```python
from build123d import *

# Parameters (mm, degrees)
SKETCH1_W           = 21.59
SKETCH1_H           = 16.51
SKETCH1_R           = 0.5
SKETCH1_W_2         = 15.24
SKETCH1_H_2         = 10.16
SKETCH1_W_3         = 9.2075
SKETCH1_H_3         = 2.38125
BOSS_EXTRUDE1_DEPTH = 1.5875
SKETCH1_3_W         = 15.24
SKETCH1_3_H         = 10.16
BOSS_EXTRUDE2_DEPTH = 3.175


with BuildPart() as part:
    # Sketch1 → Boss-Extrude1 (new body)
    # profile 1 of 4: a face of its own
    with BuildSketch(Plane.XY):
        Rectangle(SKETCH1_W, SKETCH1_H)
        with Locations((0, 7.46125)):
            Circle(SKETCH1_R, mode=Mode.SUBTRACT)
        with Locations((0, -7.46125)):
            Circle(SKETCH1_R, mode=Mode.SUBTRACT)
        Rectangle(SKETCH1_W_2, SKETCH1_H_2, mode=Mode.SUBTRACT)
    # profile 2 of 4: a face of its own
    with BuildSketch(Plane.XY):
        Rectangle(SKETCH1_W_2, SKETCH1_H_2)
    # profile 3 of 4: a face of its own
    with BuildSketch(Plane.XY):
        with Locations((0, 9.445625)):
            Rectangle(SKETCH1_W_3, SKETCH1_H_3)
    # profile 4 of 4: a face of its own
    with BuildSketch(Plane.XY):
        with Locations((0, -9.445625)):
            Rectangle(SKETCH1_W_3, SKETCH1_H_3)
    extrude(amount=BOSS_EXTRUDE1_DEPTH)

    # Sketch1_3 → Boss-Extrude2 (add)
    with BuildSketch(Plane.XY):
        Rectangle(SKETCH1_3_W, SKETCH1_3_H)
    extrude(amount=-BOSS_EXTRUDE2_DEPTH)


solid = part.part
```
Read the model definition and answer for the solid it produces. Units are mm, in the model's axes. A direction names the side the tool comes from. Give positions to 0.01 mm unless a question says otherwise; leave off trailing zeros. Write each loop counter-clockwise with the first axis right and the second up, starting at its lowest first coordinate (ties: lowest second). Pieces come first, ordered by that corner, then holes. Notation, with made-up numbers: (10, 79) - (46, 79) arc R33 cw to (46, 118) - close; hole circle Ø6 at (-35.75, 11.25). An arc over 180 degrees is marked (long way). Write item = value, one per line. Start each with the question number.
Item 1: Find section D-D (z = -1). Give the vertices of the cut face in (x, y).
Item 2: Find the intervals of material crossed by probe 1 along Y at (x, z) = (0, 0.4); probe 2 along X at (y, z) = (-0.75, -0.85); probe 3 along Z at (x, y) = (-2.5, 7.5), in increasing order. Write a range as [from, to].
Item 3: Each of these flat-tipped pins is pushed along its axis until it touches: P1, Ø1.3, axis at y = -9.5, z = 0.5, coming from the -X side; P2, Ø1, axis at x = -8, z = -1, coming from the +Y side; P3, Ø1.7, axis at x = -8, z = 1, coming from the -Y side (3 decimals). Where does it stop, or does it pass through?
Item 4: Find section A-A (x = 0). Give the vertices of the cut face in (y, z) (1 decimal), then the cut area to 3 significant figures.
Item 5: Find section B-B (y = -2.5). Give the vertices of the cut face in (x, z) (1 decimal), then the cut area to 3 significant figures.
Item 6: Find section C-C (x = -2.75). Give the vertices of the cut face in (y, z) (1 decimal).
Item 7: The mould has two halves that part along Y. Classify faces 6 (the flat face through (0, 10.636, 1)), 7 (the cylindrical face through (0.231, 7.018, 0.783)), 8 (the flat face through (0, 0, -3.175)): +Y half, -Y half, draft (parallel to the pull), parting line (faces both ways), or undercut.
Item 8: A tool of negligible diameter and unlimited length cuts with its end or side. For faces 1 (the flat face through (8, -8.255, 1)), 2 (the flat face through (0, 5.08, -2)), 3 (the flat face through (4.604, 9, 1)), 4 (the flat face through (7.62, 0, -2)), 5 (the flat face through (-4.604, -9, 1)), from which of +Z, -Z, +X, -X, +Y, -Y can it reach the whole face along a straight path? Write none if from no direction.
Response:
q1.outline = (-7.62, -5.08) - (7.62, -5.08) - (7.62, 5.08) - (-7.62, 5.08) - close
q2.probe_1 = [-10.64, -7.96], [-6.96, 6.96], [7.96, 10.64]
q2.probe_2 = [-7.62, 7.62]
q2.probe_3 = [0, 1.59]
q3.P1 = -4.6
q3.P2 = 5.08
q3.P3 = -8.255
q4.outline = (-10.6, 0) - (-8, 0) - (-8, 1.6) - (-10.6, 1.6) - close; (-7, 0) - (-5.1, 0) - (-5.1, -3.2) - (5.1, -3.2) - (5.1, 0) - (7, 0) - (7, 1.6) - (-7, 1.6) - close; (8, 0) - (10.6, 0) - (10.6, 1.6) - (8, 1.6) - close
q4.area = 62.9 mm²
q5.outline = (-10.8, 0) - (-7.6, 0) - (-7.6, -3.2) - (7.6, -3.2) - (7.6, 0) - (10.8, 0) - (10.8, 1.6) - (-10.8, 1.6) - close
q5.area = 82.7 mm²
q6.outline = (-10.6, 0) - (-5.1, 0) - (-5.1, -3.2) - (5.1, -3.2) - (5.1, 0) - (10.6, 0) - (10.6, 1.6) - (-10.6, 1.6) - close
q7.face_6 = +Y half
q7.face_7 = undercut
q7.face_8 = draft
q8.face_1 = +Z, -Z, +X, -Y
q8.face_2 = -Z, +X, -X, +Y
q8.face_3 = +Z, -Z, +X, +Y
q8.face_4 = -Z, +X, +Y, -Y
q8.face_5 = +Z, -Z, -X, -Y
